from build123d import *

# Parameters (mm, degrees)
F0_R          = 10.541
F1_DEPTH      = 25.4
F1_DEPTH_BACK = 25.4
F2_W          = 10.16
F2_H          = 5.08
F3_DEPTH      = 25.4
F3_DEPTH_BACK = 25.4
F4_R          = 3.175
F5_DEPTH      = 25.4
F5_DEPTH_BACK = 25.4


with BuildPart() as f1:
    # F0 (on Top) → F1 (new body, two sides)
    with BuildSketch(Plane.XY) as f1_sk:
        Circle(F0_R)
    extrude(amount=F1_DEPTH)
    extrude(f1_sk.sketch, amount=-F1_DEPTH_BACK)

    # F2 (on Top) → F3 (cut, two sides)
    with BuildSketch(Plane.XY) as f3_sk:
        with Locations((-0.0976234565, 2.54)):
            Rectangle(F2_W, F2_H)
    extrude(amount=-F3_DEPTH, mode=Mode.SUBTRACT)
    extrude(f3_sk.sketch, amount=F3_DEPTH_BACK, mode=Mode.SUBTRACT)

    # F4 (on Top) → F5 (cut, two sides)
    with BuildSketch(Plane.XY) as f5_sk:
        with Locations((0.0442451081, -4.3759263634)):
            Circle(F4_R)
    extrude(amount=F5_DEPTH, mode=Mode.SUBTRACT)
    extrude(f5_sk.sketch, amount=-F5_DEPTH_BACK, mode=Mode.SUBTRACT)


solid = f1.part
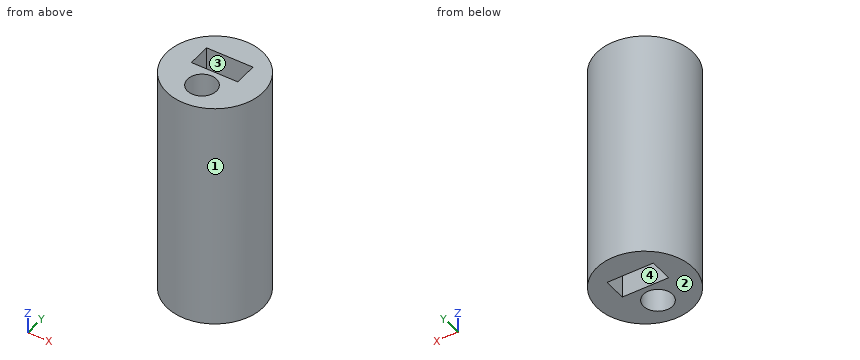
Verification items for the finished model (mm, model axes). Face numbers are marked on the shaded views. Give positions to 0.01 mm unless a question says otherwise; leave off trailing zeros. Order: outer loops, then holes, each group sorted by start corner. A loop starts at its lowest first (then second) coordinate and runs counter-clockwise, first axis right, second up. Notation, with made-up numbers: M 85,9 L 142,9 A12 ccw 142,23 Z; hole C 32.5,86.25 d9. An arc over 180 degrees is marked long. Answer as a JSON object with one key per item and string values. Group by question number.
1) Scan lines: line 1 along Y through (x, z) = (0, -14); line 2 along Y through (x, z) = (0.75, 16); line 3 along X through (y, z) = (3.5, 5). Record each from-to range of solid material in increasing order. Write a range as [from, to].
2) Cross-section at A-A (y = 3). Enter the section's corners in (x, z), then the cut area to 3 significant figures.
3) Cross-section at D-D (y = -3). Enter the section's corners in (x, z), then the cut area to 3 significant figures.
4) Mould release check, pull along X, two halves, no side actions. Record for the marked faces 1, 2, 3 and 4: released by +X, released by -X, zero draft, split by the parting line, or undercut.
5) Cross-section at B-B (x = 0). Enter the section's corners in (y, z).
6) Cross-section at C-C (z = 14). Enter the section's corners in (x, y) (3 decimals).
7) Depth check by flat-ended pin: pin 1 Ø3 at (x, z) = (-6, 15.5) entering from -Y; pin 2 Ø1 at (y, z) = (-8, -8) entering from +X; pin 3 Ø4 at (y, z) = (3.5, 3.5) entering from -X. Enter the tip coordinate at first touch or a pass-through.
Result sheet:
{
 "1": {"line 1": "y = [-10.54, -7.55], [-1.2, 0], [5.08, 10.54]", "line 2": "y = [-10.51, -7.47], [-1.28, 0], [5.08, 10.51]", "line 3": "x = [-9.94, -5.18], [4.98, 9.94]"},
 "2": {"outline": "M -10.11,-25.4 L -5.18,-25.4 L -5.18,25.4 L -10.11,25.4 Z; M 4.98,-25.4 L 10.11,-25.4 L 10.11,25.4 L 4.98,25.4 Z", "area": "511 mm2"},
 "3": {"outline": "M -10.11,-25.4 L -2.82,-25.4 L -2.82,25.4 L -10.11,25.4 Z; M 2.91,-25.4 L 10.11,-25.4 L 10.11,25.4 L 2.91,25.4 Z", "area": "736 mm2"},
 "4": {"face 1": "split by the parting line", "face 2": "zero draft", "face 3": "undercut", "face 4": "undercut"},
 "5": {"outline": "M -10.54,-25.4 L -7.55,-25.4 L -7.55,25.4 L -10.54,25.4 Z; M -1.2,-25.4 L 0,-25.4 L 0,25.4 L -1.2,25.4 Z; M 5.08,-25.4 L 10.54,-25.4 L 10.54,25.4 L 5.08,25.4 Z"},
 "6": {"outline": "C 0,0 d21.082; hole M -5.178,0 L 4.982,0 L 4.982,5.08 L -5.178,5.08 Z; hole C 0.044,-4.376 d6.35"},
 "7": {"pin 1": "stops at y = -9.53", "pin 2": "stops at x = 7.41", "pin 3": "stops at x = -10.43"}
}
